For this review, take the finished solid that the model builds, in its own axes (mm). Coordinates: 2 decimals unless noted, no trailing zeros. Write each loop counter-clockwise with the first axis right and the second up, starting at its lowest first coordinate (ties: lowest second). Pieces come first, ordered by that corner, then holes.
```python
from build123d import *

# Parameters (mm, degrees)
SKETCH1_R           = 7.5
BOSS_EXTRUDE1_DEPTH = 58


with BuildPart() as part:
    # Sketch1 → Boss-Extrude1 (new body)
    with BuildSketch(Plane.XY):
        with BuildLine():
            Line((32.5, -19), (-32.5, -19))
            Line((-32.5, -19), (-32.5, 5))
            ThreePointArc((-32.5, 5), (-15.83939444, 16.82575695), (4.16060556, 21))
            Line((4.16060556, 21), (32.5, 21))
            Line((32.5, 21), (45.490381057, 13.5))
            Line((45.490381057, 13.5), (45.490381057, -11.5))
            Line((45.490381057, -11.5), (32.5, -19))
        make_face()
        with Locations(Location((0, 0, 0), (0, 0, 180))):
            Circle(SKETCH1_R, mode=Mode.SUBTRACT)
    extrude(amount=BOSS_EXTRUDE1_DEPTH)


solid = part.part
```
Q1. Clearance check with a flat-ended pin moving along its axis: pin 1 Ø5 at (x, y) = (29.5, -14.5) entering from -Z. State where the tip first meets the part, or that it passes through.
Ans:
pin 1: stops at z = 0
Q2. Add section C-C (z = 45.5). State the section outline as (x, y) points.
Ans:
outline: (-32.5, -19) - (32.5, -19) - (45.49, -11.5) - (45.49, 13.5) - (32.5, 21) - (4.16, 21) arc R50 ccw to (-32.5, 5) - close; hole circle Ø15 at (0, 0)
Q3. Add section B-B (x = -4). State the section outline as (y, z) points.
Ans:
outline: (-19, 0) - (-6.34, 0) - (-6.34, 58) - (-19, 58) - close; (6.34, 0) - (20.33, 0) - (20.33, 58) - (6.34, 58) - close
Q4. Add section A-A (y = 3.5). State the section outline as (x, z) points, then the cut area to 3 significant figures.
Ans:
outline: (-32.5, 0) - (-6.63, 0) - (-6.63, 58) - (-32.5, 58) - close; (6.63, 0) - (45.49, 0) - (45.49, 58) - (6.63, 58) - close
area: 3,750 mm2
Q5. Draft analysis for pull direction X (two halves, no side actions). For faces 1 (the flat face through (18, 21, 29)), 2 (the cylindrical face through (-4.032, -6.324, 28.594)), 3 (the flat face through (-32.5, -7, 29)), 4 (the flat face through (39.086, -15.198, 28.594)), state which applies: +X half, -X half, draft (parallel to the pull), parting line (faces both ways), or undercut.
Ans:
face 1: draft
face 2: undercut
face 3: -X half
face 4: +X half
Q6. For probe 1 along X at (y, z) = (2.5, 44.5); probe 2 along Y at (x, z) = (0, 39); probe 3 along X at (y, z) = (-2, 51), list the stretches that pass through material, from the lowest coordinate up.
Ans:
probe 1: x = -32.5 to -7.07, 7.07 to 45.49
probe 2: y = -19 to -7.5, 7.5 to 20.83
probe 3: x = -32.5 to -7.23, 7.23 to 45.49
Q7. Add section D-D (y = -15). State the section outline as (x, z) points, then the cut area to 3 significant figures.
Ans:
outline: (-32.5, 0) - (39.43, 0) - (39.43, 58) - (-32.5, 58) - close
area: 4,170 mm2
